from build123d import *

# Parameters (mm, degrees)
F1_W     = 10
F1_H     = 3
F2_DEPTH = 3
F4_D     = 2
F6_D     = 3
F8_D     = 4.4


# Not quite as in the source:
# - a feature names something its author has since deleted; it is built from what else it names


with BuildPart() as f2:
    # F1 (on Top) → F2 (new body)
    with BuildSketch(Plane.XY):
        Polygon((-36, -70), (36, -70), (36, 70), (20, 70), (20, 63.5), (20, 60.5), (10, 60.5), (10, 63.5), (-10, 63.5), (-10, 60.5), (-20, 60.5), (-20, 63.5), (-20, 70), (-36, 70), align=None)
        with Locations((-23, -62)):
            Rectangle(F1_W, F1_H, mode=Mode.SUBTRACT)
        with Locations((23, -62)):
            Rectangle(F1_W, F1_H, mode=Mode.SUBTRACT)
        with Locations((-23, 37)):
            Rectangle(F1_W, F1_H, mode=Mode.SUBTRACT)
        with Locations((23, 37)):
            Rectangle(F1_W, F1_H, mode=Mode.SUBTRACT)
    extrude(amount=F2_DEPTH)

    # F4 (through all)
    with Locations(Plane.XY.offset(3)):
        with Locations((24, -50), (24, -42.5), (24, -35), (-24, -50), (-24, -42.5), (-24, -35), (-24, -27.5), (24, -27.5), (-24, -20), (24, -20), (-24, -12.5), (-24, -5), (-24, 2.5), (-24, 10), (-24, 17.5), (24, -12.5), (24, -5), (24, 2.5), (24, 10), (24, 17.5), (-24, 25), (24, 25)):
            Hole(F4_D / 2)

    # F6 (through all)
    with Locations(Plane(origin=(0, 0, 0), x_dir=(1, 0, 0), z_dir=(0, 0, -1))):
        with Locations((-25.5, -62), (25.5, -62), (-12, 62), (12, 62), (-12, -37), (12, -37)):
            Hole(F6_D / 2)

    # F8 (through all)
    with Locations(Plane.XY.offset(3)):
        with Locations((-12.5, -50), (12.5, -50), (-12.5, -25), (12.5, -25), (-12.5, 0), (12.5, 0), (-12.5, 25), (12.5, 25), (-12.5, 50), (12.5, 50)):
            Hole(F8_D / 2)


solid = f2.part
For this review, take the finished solid that the model builds, in its own axes (mm). A direction names the side the tool comes from. Round coordinates to 2 decimals unless told otherwise and drop trailing zeros. Order: outer loops, then holes, each group sorted by start corner. A loop starts at its lowest first (then second) coordinate and runs counter-clockwise, first axis right, second up. Notation, with made-up numbers: (15, -12) -> (38, -12) arc R26 ccw to (38, 21) -> close; hole circle Ø5 at (76.25, 25). An arc over 180 degrees is marked (long way). Put each result on its own line as item: value.
Q1. Add section A-A on y = -62. Write out the cut boundary in (x, z), plus the area to 3 significant figures.
Check result:
outline: (-36, 0) -> (-28, 0) -> (-28, 3) -> (-36, 3) -> close; (-18, 0) -> (-13.5, 0) -> (-13.5, 3) -> (-18, 3) -> close; (-10.5, 0) -> (10.5, 0) -> (10.5, 3) -> (-10.5, 3) -> close; (13.5, 0) -> (18, 0) -> (18, 3) -> (13.5, 3) -> close; (28, 0) -> (36, 0) -> (36, 3) -> (28, 3) -> close
area: 138 mm2
Q2. Mouldability with a two-part tool opening along X and no side actions: class faces 1 (the cylindrical face through (-11.675, 38.464, 1.521)), 2 (the flat face through (36, -1, 1)) as pulls with the +X half, pulls with the -X half, needs draft (parallel to the pull), parting line crosses it, or undercut.
Check result:
face 1: undercut
face 2: pulls with the +X half
Q3. Machinability: for faces 3 (the flat face through (20, 65, 1)), 4 (the flat face through (-23, 38.5, 1)), which of the approach directions +Z, -Z, +X, -X, +Y, -Y give a long, thin tool a straight path to every point of the face, cutting with its end or side? Answer none if there is none.
Check result:
face 3: +Z, -Z, +Y
face 4: +Z, -Z
Q4. For probe 1 along X at (y, z) = (37, 2.4); probe 2 along Y at (x, z) = (-25.5, 0.7); probe 3 along X at (y, z) = (36, 2.4), list the stretches that pass through material, from the lowest coordinate up. Write a range as [from, to].
Check result:
probe 1: [-36, -28], [-18, -13.5], [-10.5, 10.5], [13.5, 18], [28, 36]
probe 2: [-70, -63.5], [-60.5, 35.5], [38.5, 60.5], [63.5, 70]
probe 3: [-36, -28], [-18, -13.12], [-10.88, 10.88], [13.12, 18], [28, 36]
Q5. Add section B-B on x = 12. State how many separate pieces and enclosed holes the cut face has, plus the area to 3 significant figures.
Check result:
separate pieces: 8
enclosed holes: 0
area: 309 mm2
Q6. Insertion check: pin 1 Ø2.5 at (x, y) = (-12.5, 0) entering from +Z; pin 2 Ø1.5 at (x, z) = (13, 1) entering from +Y. Each pin has a flat end and moves straight along its axis. Give the tip position at first contact, or say it passes through.
Check result:
pin 1: through
pin 2: y = 60.5
